The drawing under review shows one solid part. Ordinate dimensions are in mm from its lowest x, y, z. A direction names the side the tool comes from. Round coordinates to 2 decimals unless told otherwise and drop trailing zeros. Order: outer loops, then holes, each group sorted by start corner. A loop starts at its lowest first (then second) coordinate and runs counter-clockwise, first axis right, second up. Notation, with made-up numbers: (30.5, -18) - (80.5, -18) arc R21 ccw to (80.5, -5) - close; hole circle Ø2 at (10.25, -10.5). An arc over 180 degrees is marked (long way). Answer as a JSON object with one key per item and string values. Group by question number.
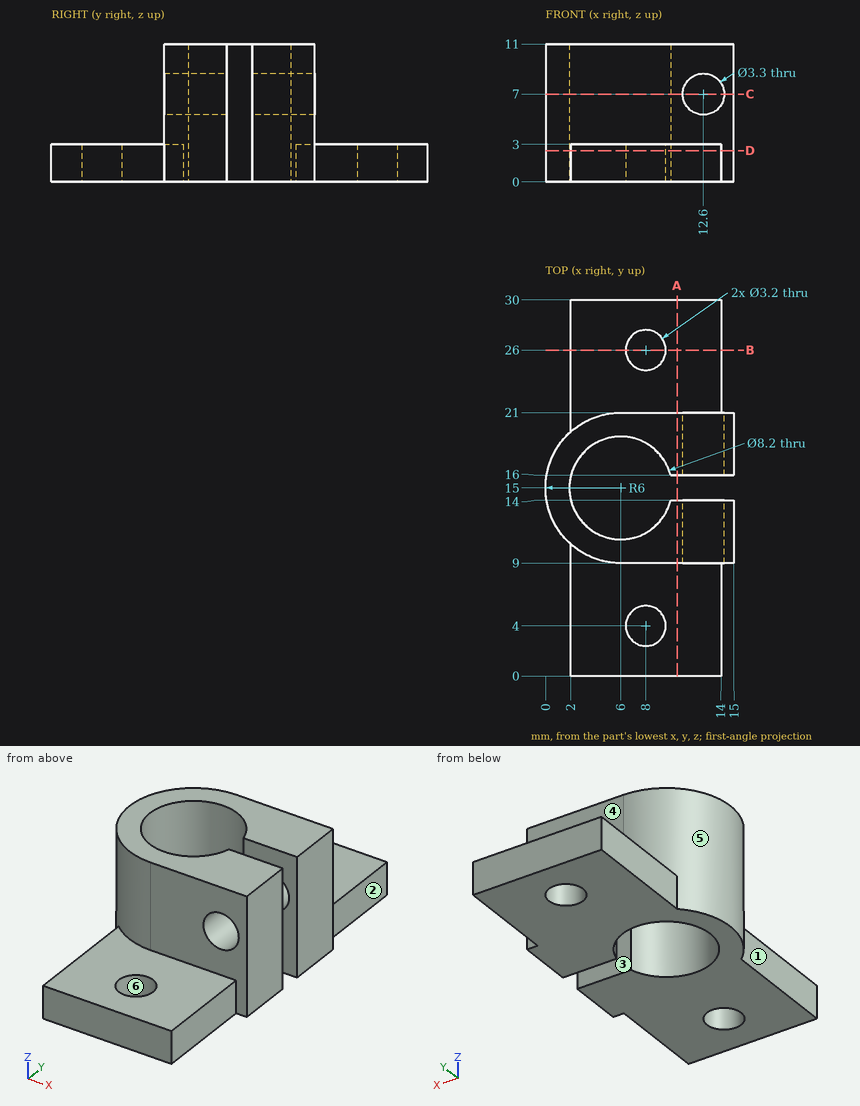
1. Tool access review of the marked faces 1, 2 and 3: name each direction out of +Z, -Z, +X, -X, +Y, -Y from which nothing blocks a thin tool from reaching the whole face with its end or side.
2. Clearance check with flat-ended pins moving along their axes: P1, Ø1.5, axis at x = 2, y = 11.5, coming from the -Z side; P2, Ø5.5, axis at x = 12.6, z = 7, coming from the -Y side; P3, Ø2.5, axis at x = 8, y = 4, coming from the -Z side; P4, Ø1.5, axis at y = 7, z = 1.5, coming from the -X side. State where each tip first meets the part, or that it passes through.
3. Take a section at C-C, the plane z = 7. Give the boundary of the cut face in (x, y), then the cut area to 3 significant figures.
4. Take a section at A-A, the plane x = 10.5. Give the boundary of the cut face in (y, z), then the cut area to 3 significant figures.
5. Take a section at B-B, the plane y = 26. Give the boundary of the cut face in (x, z), then the cut area to 3 significant figures.
6. Mouldability with a two-part tool opening along X and no side actions: class the marked faces 4, 5 and 6 as pulls with the +X half, pulls with the -X half, needs draft (parallel to the pull), parting line crosses it, or undercut.
7. Take a section at D-D, the plane z = 2.5. Give the boundary of the cut face in (x, y).
8. To check wall thickness, follow line 1 (Y direction, x = 6, z = 5); line 2 (Y direction, x = 12.75, z = 1.75); line 3 (Z direction, x = 12.6, y = 17.1). State the ranges of each line that lie inside material, in increasing order. Write a range as from..to.
Response values:
{
 "1": {"face 1": "+Z, -Z, -X, -Y", "face 2": "+Z, -Z, +X, +Y", "face 3": "+Z, -Z, +X"},
 "2": {"P1": "z = 0", "P2": "y = 9", "P3": "through", "P4": "x = 2"},
 "3": {"outline": "(6, 9) - (10.95, 9) - (10.95, 14) - (9.98, 14) arc R4.1 cw (long way) to (9.98, 16) - (10.95, 16) - (10.95, 21) - (6, 21) arc R6 ccw to start; (14.25, 9) - (15, 9) - (15, 14) - (14.25, 14) - close; (14.25, 16) - (15, 16) - (15, 21) - (14.25, 21) - close", "area": "68.9 mm2"},
 "4": {"outline": "(0, 0) - (14, 0) - (14, 11) - (9, 11) - (9, 3) - (0, 3) - close; (16, 0) - (30, 0) - (30, 3) - (21, 3) - (21, 11) - (16, 11) - close", "area": "164 mm2"},
 "5": {"outline": "(2, 0) - (6.4, 0) - (6.4, 3) - (2, 3) - close; (9.6, 0) - (14, 0) - (14, 3) - (9.6, 3) - close", "area": "26.4 mm2"},
 "6": {"face 4": "needs draft", "face 5": "pulls with the -X half", "face 6": "undercut"},
 "7": {"outline": "(2, 0) - (14, 0) - (14, 9) - (15, 9) - (15, 14) - (9.98, 14) arc R4.1 cw (long way) to (9.98, 16) - (15, 16) - (15, 21) - (14, 21) - (14, 30) - (2, 30) - (2, 19.47) arc R6 ccw to (2, 10.53) - close; hole circle Ø3.2 at (8, 4); hole circle Ø3.2 at (8, 26)"},
 "8": {"line 1": "9..10.9, 19.1..21", "line 2": "0..14, 16..30", "line 3": "0..5.35, 8.65..11"}
}
